Build history of the part. All positions in model axes, mm. Round coordinates to 2 decimals unless told otherwise and drop trailing zeros. Order: outer loops, then holes, each group sorted by start corner. A loop starts at its lowest first (then second) coordinate and runs counter-clockwise, first axis right, second up. Notation, with made-up numbers: (14, 30) -> (35, 30) arc R10 ccw to (35, 41) -> close; hole circle Ø9 at (22.5, -39). An arc over 180 degrees is marked (long way). Answer as a JSON object with one key per item and string values.
from build123d import *

# Parameters (mm, degrees)
SKETCH1_W           = 22.4
SKETCH1_H           = 27.2
SKETCH1_R           = 1.6
SKETCH1_R_2         = 0.5
BOSS_EXTRUDE1_DEPTH = 1.5


with BuildPart() as part:
    # Sketch1 → Boss-Extrude1 (new body)
    with BuildSketch(Plane(origin=(0, 0, 0), x_dir=(1, 0, 0), z_dir=(0, 1, 0))):
        Rectangle(SKETCH1_W, SKETCH1_H)
        with Locations((7.2, 9.6)):
            Circle(SKETCH1_R, mode=Mode.SUBTRACT)
        with Locations((-7.2, 9.6)):
            Circle(SKETCH1_R, mode=Mode.SUBTRACT)
        with Locations((-7.2, -9.6)):
            Circle(SKETCH1_R, mode=Mode.SUBTRACT)
        with Locations((-1.7, -9.9)):
            Circle(SKETCH1_R_2, mode=Mode.SUBTRACT)
        with Locations((1.7, -9.9)):
            Circle(SKETCH1_R_2, mode=Mode.SUBTRACT)
        with Locations((7.2, -9.6)):
            Circle(SKETCH1_R, mode=Mode.SUBTRACT)
    extrude(amount=-BOSS_EXTRUDE1_DEPTH)


solid = part.part
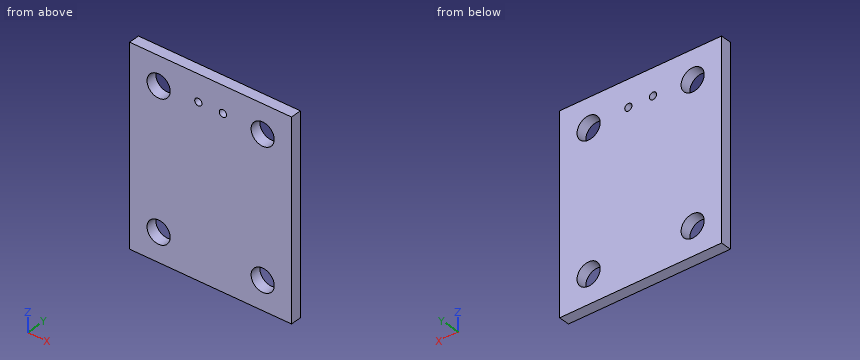
1) Cut at D-D, the plane x = 1.7. Give the cut face in (y, z), plus the area to 3 significant figures.
Checked values:
{"outline": "(-1.5, -13.6) -> (0, -13.6) -> (0, 9.4) -> (-1.5, 9.4) -> close; (-1.5, 10.4) -> (0, 10.4) -> (0, 13.6) -> (-1.5, 13.6) -> close", "area": "39.3 mm²"}
2) Cut at B-B, the plane y = -0.5. Give the cut face in (x, z).
Checked values:
{"outline": "(-11.2, -13.6) -> (11.2, -13.6) -> (11.2, 13.6) -> (-11.2, 13.6) -> close; hole circle Ø3.2 at (-7.2, -9.6); hole circle Ø3.2 at (-7.2, 9.6); hole circle Ø1 at (-1.7, 9.9); hole circle Ø1 at (1.7, 9.9); hole circle Ø3.2 at (7.2, -9.6); hole circle Ø3.2 at (7.2, 9.6)"}
3) Probe L1, parallel to X at y = -1.1, z = -9.6; L2, parallel to X at y = -0.7, z = 9.9; L3, parallel to Z at x = 7.2, y = -0.9. List the from-to ranges inside material, lowest first. Write a range as from..to.
Checked values:
{"L1": "x = -11.2..-8.8, -5.6..5.6, 8.8..11.2", "L2": "x = -11.2..-8.77, -5.63..-2.2, -1.2..1.2, 2.2..5.63, 8.77..11.2", "L3": "z = -13.6..-11.2, -8..8, 11.2..13.6"}
4) Flat gauge pin, fed straight in: pin 1 Ø5 at (x, z) = (-8, 4) entering from +Y. Where does the tip first touch, or does it go through?
Checked values:
{"pin 1": "stops at y = 0"}
5) Cut at A-A, the plane x = 7.2. Give the cut face in (y, z).
Checked values:
{"outline": "(-1.5, -13.6) -> (0, -13.6) -> (0, -11.2) -> (-1.5, -11.2) -> close; (-1.5, -8) -> (0, -8) -> (0, 8) -> (-1.5, 8) -> close; (-1.5, 11.2) -> (0, 11.2) -> (0, 13.6) -> (-1.5, 13.6) -> close"}
6) Cut at C-C, the plane z = 9.9. Give the cut face in (x, y).
Checked values:
{"outline": "(-11.2, -1.5) -> (-8.77, -1.5) -> (-8.77, 0) -> (-11.2, 0) -> close; (-5.63, -1.5) -> (-2.2, -1.5) -> (-2.2, 0) -> (-5.63, 0) -> close; (-1.2, -1.5) -> (1.2, -1.5) -> (1.2, 0) -> (-1.2, 0) -> close; (2.2, -1.5) -> (5.63, -1.5) -> (5.63, 0) -> (2.2, 0) -> close; (8.77, -1.5) -> (11.2, -1.5) -> (11.2, 0) -> (8.77, 0) -> close"}
